from build123d import *

# Parameters (mm, degrees)
F1_DEPTH = 552
F2_W     = 12
F2_H     = 70
F3_DEPTH = 520
F4_W     = 595
F4_H     = 125
F5_DEPTH = 20


with BuildPart() as f1:
    # F0 (on Front) → F1 (new body)
    with BuildSketch(Plane.XZ):
        Polygon((260, 55), (260, 3), (-260, 3), (-260, 55), (-272, 55), (-272, -15), (-260, -15), (-260, -3), (260, -3), (260, -15), (272, -15), (272, 55), align=None)
    extrude(amount=F1_DEPTH)

    # F2 (on face) → F3 (join)
    with BuildSketch(Plane(origin=(260, 0, 0), x_dir=(0, -1, 0), z_dir=(-1, 0, 0))):
        with Locations((6, 20)):
            Rectangle(F2_W, F2_H)
        with Locations((546, 20)):
            Rectangle(F2_W, F2_H)
    extrude(amount=F3_DEPTH)

    # F4 (on face) → F5 (join)
    with BuildSketch(Plane.XZ.offset(552)):
        with Locations((0, 14.5)):
            Rectangle(F4_W, F4_H)
    extrude(amount=F5_DEPTH)


solid = f1.part
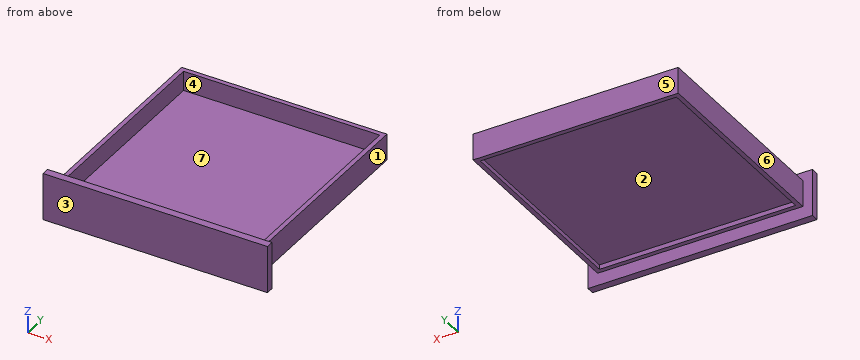
Read the model definition and answer for the solid it produces. Units are mm, in the model's axes. Face numbers are marked on the shaded views. A direction names the side the tool comes from. Round coordinates to 2 decimals unless told otherwise and drop trailing zeros. Write each loop counter-clockwise with the first axis right and the second up, starting at its lowest first coordinate (ties: lowest second). Pieces come first, ordered by that corner, then holes.
Q1. Flat-ended cylindrical pins translate along their axes: P1, Ø1, axis at y = -344, z = 35, coming from the +X side; P2, Ø3.5, axis at y = -209.5, z = -11, coming from the -X side; P3, Ø10, axis at x = 103.5, y = -283, coming from the +Z side. Find the tip coordinate at first contact, or state that the pin passes through.
Values:
P1: stops at x = 272
P2: stops at x = -272
P3: stops at z = 3
Q2. Straight lines are drawn through the part: line 1 (X direction, y = -421, z = 42); line 2 (Y direction, x = 246, z = 41.5); line 3 (Z direction, x = -113.5, y = -234.5). For each, find the intervals that lie inside material, in ascending order.
Values:
line 1: x = -272 to -260, 260 to 272
line 2: y = -572 to -540, -12 to 0
line 3: z = -3 to 3
Q3. The mould has two halves that part along X. Classify the marked faces 4, 5, 6 and 7: released by +X, released by -X, zero draft, split by the parting line, or undercut.
Values:
face 4: undercut
face 5: zero draft
face 6: released by -X
face 7: undercut
Q4. Find section C-C on y = -216.5. Determine the outline of the cut face in (x, z).
Values:
outline: (-272, -15) - (-260, -15) - (-260, -3) - (260, -3) - (260, -15) - (272, -15) - (272, 55) - (260, 55) - (260, 3) - (-260, 3) - (-260, 55) - (-272, 55) - close
Q5. Find section B-B on x = -153. Determine the outline of the cut face in (y, z).
Values:
outline: (-572, -48) - (-552, -48) - (-552, -15) - (-540, -15) - (-540, -3) - (-12, -3) - (-12, -15) - (0, -15) - (0, 55) - (-12, 55) - (-12, 3) - (-540, 3) - (-540, 55) - (-552, 55) - (-552, 77) - (-572, 77) - close
Q6. Find section D-D on z = -27. Determine the outline of the cut face in (x, y).
Values:
outline: (-297.5, -572) - (297.5, -572) - (297.5, -552) - (-297.5, -552) - close
Q7. A tool of negligible diameter and unlimited length cuts with its end or side. For the marked faces 1, 2 and 3, from which of +Z, -Z, +X, -X, +Y, -Y can it reach the whole face along a straight path? Write none if from no direction.
Values:
face 1: +Z, -Z, +X, +Y
face 2: -Z
face 3: +Z, -Z, +X, -X, -Y
Q8. Find section A-A on z = 16. Determine the outline of the cut face in (x, y), and give its area (3 significant figures).
Values:
outline: (-297.5, -572) - (297.5, -572) - (297.5, -552) - (272, -552) - (272, 0) - (-272, 0) - (-272, -552) - (-297.5, -552) - close; hole (-260, -540) - (260, -540) - (260, -12) - (-260, -12) - close
area: 37,600 mm2
